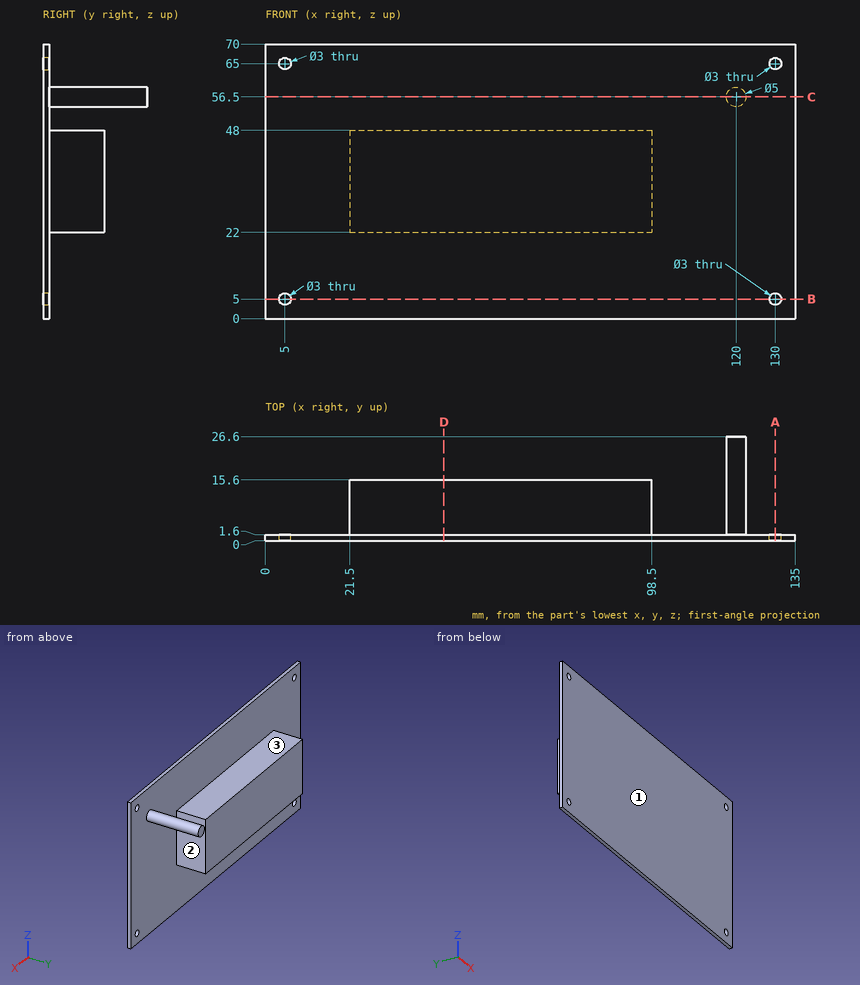
Drawing for the job (mm, zero at the part's lowest x, y, z). A direction names the side the tool comes from. Give positions to 0.01 mm unless a question says otherwise; leave off trailing zeros. Loops run counter-clockwise (first coordinate to the right, second up) from the corner with the lowest first, then second, coordinate; pieces in that order, holes last.
1) 3-axis set-ups, long thin cutter, end or side, ignore diameter. For the marked faces 1, 2 and 3: which of +Z, -Z, +X, -X, +Y, -Y reach the whole face in a straight line?
Values follow:
face 1: +Z, -Z, +X, -X, -Y
face 2: +Z, -Z, +X, +Y
face 3: +Z, +X, -X, +Y
2) Band-saw the part on A-A on x = 130. List the corners of the cut face in (y, z).
Values follow:
outline: (0, 0) - (1.6, 0) - (1.6, 3.5) - (0, 3.5) - close; (0, 6.5) - (1.6, 6.5) - (1.6, 63.5) - (0, 63.5) - close; (0, 66.5) - (1.6, 66.5) - (1.6, 70) - (0, 70) - close
3) Band-saw the part on B-B on z = 5. List the corners of the cut face in (x, y), then the cut area to 3 significant figures.
Values follow:
outline: (0, 0) - (3.5, 0) - (3.5, 1.6) - (0, 1.6) - close; (6.5, 0) - (128.5, 0) - (128.5, 1.6) - (6.5, 1.6) - close; (131.5, 0) - (135, 0) - (135, 1.6) - (131.5, 1.6) - close
area: 206 mm2
4) Band-saw the part on D-D on x = 45.5. List the corners of the cut face in (y, z).
Values follow:
outline: (0, 0) - (1.6, 0) - (1.6, 22) - (15.6, 22) - (15.6, 48) - (1.6, 48) - (1.6, 70) - (0, 70) - close
5) Drop flat-ended pins along their axis: P1, Ø8, axis at x = 119, y = 12.5, coming from the +Z side; P2, Ø11, axis at x = 51.5, y = 11, coming from the -Z side; P3, Ø10, axis at y = 10, z = 59.5, coming from the +X side. Give the stop position or say it passes through.
Values follow:
P1: stops at z = 59
P2: stops at z = 22
P3: stops at x = 122.5
6) Band-saw the part on C-C on z = 56.5. List the corners of the cut face in (x, y).
Values follow:
outline: (0, 0) - (135, 0) - (135, 1.6) - (122.5, 1.6) - (122.5, 26.6) - (117.5, 26.6) - (117.5, 1.6) - (0, 1.6) - close
7) Probe line 1 along Z through (x, y) = (130, 0.95); line 2 along X through (y, z) = (0.9, 65); line 3 along Y through (x, z) = (92, 61). List the from-to ranges inside material, lowest first.
Values follow:
line 1: z = 0 to 3.5, 6.5 to 63.5, 66.5 to 70
line 2: x = 0 to 3.5, 6.5 to 128.5, 131.5 to 135
line 3: y = 0 to 1.6
